Can you work these out from the model? Positions are in its coordinate system, mm. A direction names the side the tool comes from. Give positions to 0.01 mm unless a question says otherwise; leave off trailing zeros. Order: outer loops, then holes, each group sorted by start corner. A loop starts at its lowest first (then second) coordinate and runs counter-clockwise, first axis right, second up. Notation, with made-up numbers: (10, 9.25) - (33, 9.25) arc R26 cw to (33, 24.25) - close; hole circle Ø8 at (69.25, -10). An arc over 180 degrees is marked (long way). Use one line per item in the form item = value. Start each with the question number.
1) Suppose I cut it at A-A, the plane y = 6.25. Write out the boundary of the cut face in (x, z) (3 decimals), and give its area (3 significant figures).
2) We'd pull the mould along X, two halves only. Please class faces 1 (the flat face through (160, 12.7, -3)), 2 (the flat face through (246, 8, -6.35)), 3 (the flat face through (2, 2, -13)), 4 (the flat face through (243.84, 8, -13)): released by +X, released by -X, zero draft, split by the parting line, or undercut.
3) Suppose I cut it at B-B, the plane z = -14.5. Write out the boundary of the cut face in (x, y) (3 decimals).
4) Please list where these lines run through material, in increasing order: probe 1 along X at (y, z) = (4.5, -6.5) (3 decimals); probe 2 along Z at (x, y) = (163.5, 3.25); probe 3 along X at (y, z) = (2.75, -15) (3 decimals).
5) Suppose I cut it at C-C, the plane x = 73. Write out the boundary of the cut face in (y, z), and give its area (3 significant figures).
6) Which directions (+Z, -Z, +X, -X, +Y, -Y) give clear straight access to the entire face, cutting with the end or side of a thin tool? Please do faces 5 (the flat face through (248.92, 8, -13)), 6 (the flat face through (254, 6, -13)).
7) For pin 1 (1.5 mm diameter, centred on x = 229, z = -12, fed in from +Y); pin 2 (2 mm diameter, centred on y = 8, z = -9.5, fed in from -X) (3 decimals); pin 3 (1 mm diameter, centred on y = 3.5, z = -14, fed in from -X), each with a flat end and sliding along its axis, tell me the tip position at first contact or that it passes through.
```python
from build123d import *

# Parameters (mm, degrees)
SKETCH1_W          = 254
SKETCH1_H          = 25.4
BASE_EXTRUDE_DEPTH = 12.7
SKETCH3_W          = 215.9
SKETCH3_H          = 17.526
PIECE_CUT_DEPTH    = 10.16
CORNER_CUT_DEPTH   = 256.582569828
SKETCH6_W          = 5.08
SKETCH6_H          = 12.7
PEG_CUT_DEPTH      = 10.16


with BuildPart() as part:
    # Sketch1 → Base Extrude (new body)
    with BuildSketch(Plane(origin=(0, 0, 0), x_dir=(1, 0, 0), z_dir=(0, 1, 0))):
        with Locations((127, 12.7)):
            Rectangle(SKETCH1_W, SKETCH1_H)
    extrude(amount=BASE_EXTRUDE_DEPTH)

    # Sketch3 → Piece Cut (cut)
    with BuildSketch(Plane(origin=(0, 12.7, 0), x_dir=(1, 0, 0), z_dir=(0, 1, 0))):
        with Locations((111.125, 12.7)):
            Rectangle(SKETCH3_W, SKETCH3_H)
    extrude(amount=-PIECE_CUT_DEPTH, mode=Mode.SUBTRACT)

    # Sketch4 → Corner Cut (cut, through all)
    with BuildSketch(Plane(origin=(0, 0, -25.4), x_dir=(-1, 0, 0), z_dir=(0, 0, -1))):
        Polygon((0, 0), (-12.7, 12.7), (0, 12.7), align=None)
    extrude(amount=-CORNER_CUT_DEPTH, mode=Mode.SUBTRACT)

    # Sketch6 → Peg Cut (cut)
    with BuildSketch(Plane(origin=(0, 12.7, 0), x_dir=(1, 0, 0), z_dir=(0, 1, 0))):
        with Locations((229.235, 12.7)):
            Rectangle(SKETCH6_W, SKETCH6_H)
        with Locations((246.38, 12.7)):
            Rectangle(SKETCH6_W, SKETCH6_H)
    extrude(amount=-PEG_CUT_DEPTH, mode=Mode.SUBTRACT)


solid = part.part
```
Result sheet:
q1.outline = (6.25, -25.4) - (254, -25.4) - (254, 0) - (6.25, 0) - (6.25, -3.937) - (219.075, -3.937) - (219.075, -21.463) - (6.25, -21.463) - close; hole (226.695, -19.05) - (231.775, -19.05) - (231.775, -6.35) - (226.695, -6.35) - close; hole (243.84, -19.05) - (248.92, -19.05) - (248.92, -6.35) - (243.84, -6.35) - close
q1.area = 2,430 mm²
q2.face_1 = zero draft
q2.face_2 = undercut
q2.face_3 = released by -X
q2.face_4 = undercut
q3.outline = (0, 0) - (254, 0) - (254, 12.7) - (248.92, 12.7) - (248.92, 2.54) - (243.84, 2.54) - (243.84, 12.7) - (231.775, 12.7) - (231.775, 2.54) - (226.695, 2.54) - (226.695, 12.7) - (219.075, 12.7) - (219.075, 2.54) - (3.175, 2.54) - (3.175, 3.175) - close
q4.probe_1 = 219.075 to 226.695, 231.775 to 243.84, 248.92 to 254
q4.probe_2 = -25.4 to -21.46, -3.94 to 0
q4.probe_3 = 2.75 to 3.175, 219.075 to 226.695, 231.775 to 243.84, 248.92 to 254
q5.outline = (0, -25.4) - (12.7, -25.4) - (12.7, -21.46) - (2.54, -21.46) - (2.54, -3.94) - (12.7, -3.94) - (12.7, 0) - (0, 0) - close
q5.area = 145 mm²
q6.face_5 = +Y
q6.face_6 = +Z, -Z, +X, +Y, -Y
q7.pin_1 = 2.54
q7.pin_2 = 219.075
q7.pin_3 = 3
